from build123d import *

# Parameters (mm, degrees)
BOSS_EXTRUDE1_DEPTH = 40
SKETCH2_W           = 180
SKETCH2_H           = 50
CUT_EXTRUDE1_DEPTH  = 171.293863659
SKETCH3_R           = 17.5
BOSS_EXTRUDE2_DEPTH = 3
SKETCH4_R           = 30
BOSS_EXTRUDE3_DEPTH = 10
SKETCH5_R           = 25
BOSS_EXTRUDE4_DEPTH = 3
FILLET1_R           = 100
FILLET2_R           = 10
FILLET3_R           = 5


with BuildPart() as part:
    # Sketch1 → Boss-Extrude1 (new, symmetric)
    with BuildSketch(Plane.XY):
        with BuildLine():
            Line((0, 0), (94.268250808, 0))
            Line((94.268250808, 0), (125.20944533, 5.45576741))
            ThreePointArc((125.20944533, 5.45576741), (150, 35), (125.20944533, 64.54423259))
            Line((125.20944533, 64.54423259), (94.268250808, 70))
            Line((94.268250808, 70), (0, 70))
            Line((0, 70), (0, 0))
        make_face()
    extrude(amount=BOSS_EXTRUDE1_DEPTH, both=True)

    # Sketch2 → Cut-Extrude1 (cut, through all)
    with BuildSketch(Plane(origin=(0, 0, 0), x_dir=(1, 0, 0), z_dir=(0, 1, 0))):
        with Locations((110, 0)):
            Rectangle(SKETCH2_W, SKETCH2_H)
    extrude(amount=CUT_EXTRUDE1_DEPTH, mode=Mode.SUBTRACT)

    # Sketch3 → Boss-Extrude2 (add)
    with BuildSketch(Plane.XY.offset(-25)):
        with Locations((120, 35)):
            Circle(SKETCH3_R)
    boss_extrude2 = extrude(amount=BOSS_EXTRUDE2_DEPTH)

    # Mirror1: Boss-Extrude2 across plane
    add(boss_extrude2.mirror(Plane.XY))

    # Sketch4 → Boss-Extrude3 (add)
    with BuildSketch(Plane.ZY):
        with Locations((0, 35)):
            Circle(SKETCH4_R)
    extrude(amount=BOSS_EXTRUDE3_DEPTH)

    # Sketch5 → Boss-Extrude4 (add)
    with BuildSketch(Plane.ZY.offset(10)):
        with Locations((0, 35)):
            Circle(SKETCH5_R)
    extrude(amount=BOSS_EXTRUDE4_DEPTH)

    # Fillet1
    fillet1_edges = [part.edges().sort_by_distance(p)[0] for p in [
        (94.268250808, 70, 32.5),
        (94.268250808, 0, 32.5),
        (94.268250808, 70, -32.5),
        (94.268250808, 0, -32.5),
    ]]
    fillet(fillet1_edges, radius=FILLET1_R)

    # Fillet2
    fillet2_edges = [part.edges().sort_by_distance(p)[0] for p in [
        (20, 35, 25),
        (20, 35, -25),
    ]]
    fillet(fillet2_edges, radius=FILLET2_R)

    # Fillet3
    fillet3_edges = [part.edges().sort_by_distance(p)[0] for p in [
        (0, 70, 0),
        (0, 0, 0),
        (150, 35, 40),
        (114.046823776, 66.512503946, 40),
        (150, 35, 25),
        (114.046823776, 3.487496054, 25),
        (150, 35, -25),
        (114.046823776, 66.512503946, -25),
        (0, 35, 40),
        (114.046823776, 3.487496054, -25),
        (114.046823776, 3.487496054, -40),
        (114.046823776, 66.512503946, -40),
        (42.759692228, 70, -40),
        (94.23495873, 69.619469809, -40),
        (94.23495873, 0.380530191, -40),
        (57.759692228, 0, -25),
        (150, 35, -40),
        (42.759692228, 0, 40),
        (57.759692228, 70, -25),
        (94.23495873, 69.619469809, -25),
        (94.23495873, 0.380530191, -25),
        (114.046823776, 3.487496054, 40),
        (114.046823776, 66.512503946, 25),
        (94.23495873, 69.619469809, 25),
        (94.23495873, 0.380530191, 25),
        (42.759692228, 70, 40),
        (94.23495873, 69.619469809, 40),
        (94.23495873, 0.380530191, 40),
        (42.759692228, 0, -40),
        (0, 35, -40),
        (20, 0, 0),
        (20, 70, 0),
        (57.759692228, 0, 25),
        (57.759692228, 70, 25),
        (22.928932188, 0, -22.071067812),
        (22.928932188, 70, -22.071067812),
        (22.928932188, 0, 22.071067812),
        (22.928932188, 70, 22.071067812),
    ]]
    fillet(fillet3_edges, radius=FILLET3_R - 0.0001)  # a hair under: the kernel refuses the full size


solid = part.part
Model file for the job. Use its own axes, mm. A direction names the side the tool comes from. Give positions to 0.01 mm unless a question says otherwise; leave off trailing zeros. Loops run counter-clockwise (first coordinate to the right, second up) from the corner with the lowest first, then second, coordinate; pieces in that order, holes last. Notation, with made-up numbers: (34, 15) - (53, 15) arc R13 cw to (53, 36) - close; hole circle Ø11 at (34, 30). An arc over 180 degrees is marked (long way). Use one line per item in the form item = value.
(1) 3-axis set-ups, long thin cutter, end or side, ignore diameter. For faces 1 (the face through (19, 68, 0)), 2 (the face through (-10, 60, -7)), 3 (the face through (22.85, 35.42, -21.99)), 4 (the face through (57, 2, -26)): which of +Z, -Z, +X, -X, +Y, -Y reach the whole face in a straight line?
Determined:
face_1 = +X, +Y
face_2 = -X
face_3 = +Y, -Y
face_4 = +X, -Y
(2) Drop flat-ended pins along their axis: P1, Ø24, axis at y = 24, z = 5, coming from the +X side; P2, Ø1.5, axis at y = 24, z = 27.5, coming from the +X side; P3, Ø10, axis at y = 29.5, z = -29, coming from the +X side. Give the stop position or say it passes through.
Determined:
P1 = 20.2
P2 = 147.68
P3 = 149.99
(3) Drill centre lines: L1, parallel to Z at x = 95.5, y = 56.5; L2, parallel to X at y = 52, z = -14.5; L3, parallel to X at y = 6, z = -13. Where is each one in solid material? Low to high.
Determined:
L1 = -40 to -25, 25 to 40
L2 = -13 to 20
L3 = 0 to 20
(4) Pull direction Z, two halves, no side cores. Call faces 5 (the face through (113.629, 4.941, -26.426)), 6 (the face through (113.629, 65.059, 38.574)), 7 (the face through (149.994, 34.414, 32.535)): pulls with the +Z half, pulls with the -Z half, needs draft (parallel to the pull), parting line crosses it, or undercut.
Determined:
face_5 = undercut
face_6 = pulls with the +Z half
face_7 = needs draft
(5) Cut at A-A (x = 62). Give the cut face in (y, z), then the cut area to 3 significant figures.
Determined:
outline = (0, -35) arc R5 ccw to (5, -40) - (65, -40) arc R5 ccw to (70, -35) - (70, -30) arc R5 ccw to (65, -25) - (5, -25) arc R5 ccw to (0, -30) - close; (0, 30) arc R5 ccw to (5, 25) - (65, 25) arc R5 ccw to (70, 30) - (70, 35) arc R5 ccw to (65, 40) - (5, 40) arc R5 ccw to (0, 35) - close
area = 2,060 mm^2
